Verification items for this drawing (mm, ordinates from the low corner). Round coordinates to 2 decimals unless told otherwise and drop trailing zeros. Order: outer loops, then holes, each group sorted by start corner. A loop starts at its lowest first (then second) coordinate and runs counter-clockwise, first axis right, second up. Notation, with made-up numbers: (74.25, 81.5) -> (105.25, 81.5) arc R26 cw to (105.25, 95.5) -> close; hole circle Ø8 at (-7, 34). An arc over 180 degrees is marked (long way). Return JSON: item names as keys, results as strings. Group by question number.
Item 1: Sectioned sample at C-C on y = 11. Record the cut outline in (x, z).
Item 2: Draft check along Z on the marked faces 1, 2 and 3. Enter one of: pulls with the +Z half, pulls with the -Z half, needs draft (parallel to the pull), parting line crosses it, or undercut.
Item 3: Depth check by flat-ended pin: pin 1 Ø2 at (x, y) = (44, 9) entering from +Z; pin 2 Ø8 at (x, z) = (81, 79.5) entering from -Y; pin 3 Ø23.5 at (x, z) = (45, 45) entering from -Y; pin 4 Ø3 at (x, z) = (58, 72) entering from -Y. Enter the tip coordinate at first touch or a pass-through.
Item 4: Sectioned sample at A-A on x = 45. Record the cut outline in (y, z).
Item 5: Sectioned sample at D-D on z = 14. Record the cut outline in (x, y).
Item 6: Scan lines: probe 1 along X at (y, z) = (26.45, 45); probe 2 along Y at (x, z) = (72, 51.5); probe 3 along X at (y, z) = (19.25, 45). Record each from-to range of solid material in increasing order. Write a range as from..to.
Item 7: Sectioned sample at B-B on z = 45. Record the cut outline in (x, y), plus the area to 3 significant figures.
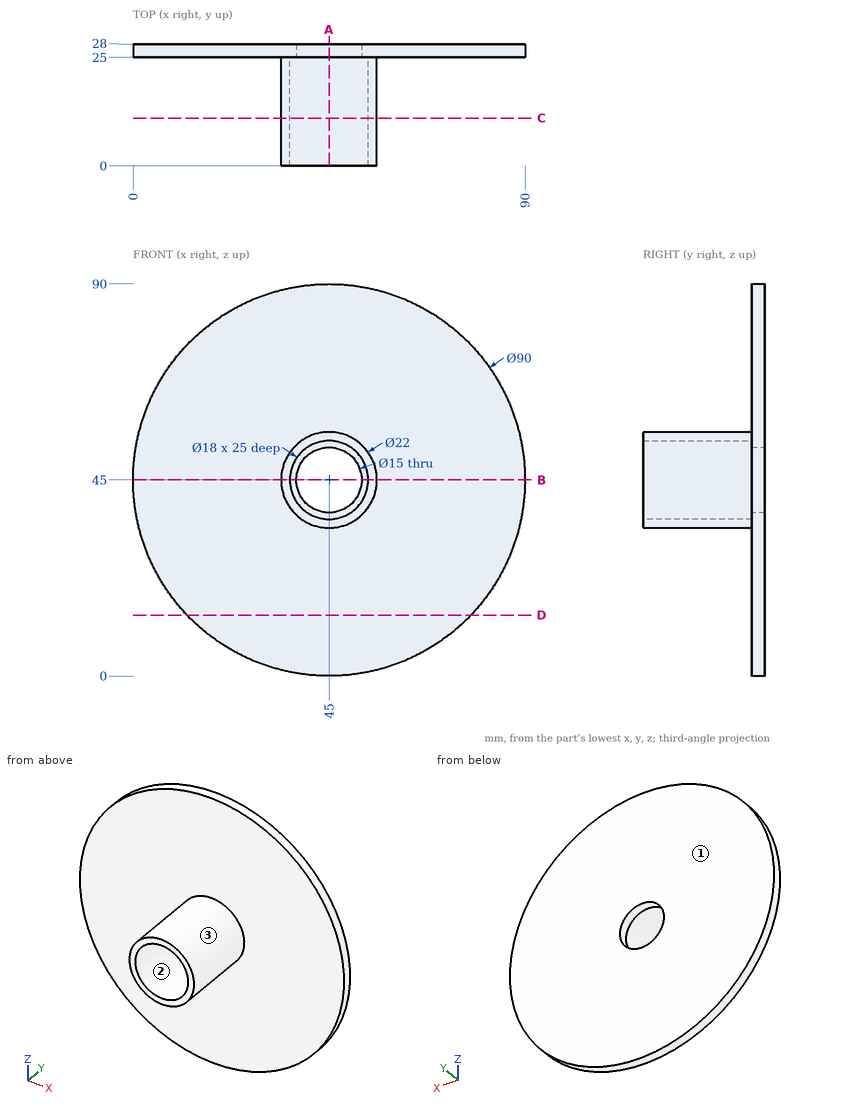
Recorded:
{
 "1": {"outline": "circle Ø22 at (45, 45); hole circle Ø18 at (45, 45)"},
 "2": {"face 1": "needs draft", "face 2": "undercut", "face 3": "parting line crosses it"},
 "3": {"pin 1": "z = 56", "pin 2": "through", "pin 3": "y = 0", "pin 4": "y = 25"},
 "4": {"outline": "(0, 34) -> (25, 34) -> (25, 0) -> (28, 0) -> (28, 37.5) -> (25, 37.5) -> (25, 36) -> (0, 36) -> close; (0, 54) -> (25, 54) -> (25, 52.5) -> (28, 52.5) -> (28, 90) -> (25, 90) -> (25, 56) -> (0, 56) -> close"},
 "5": {"outline": "(12.38, 25) -> (77.62, 25) -> (77.62, 28) -> (12.38, 28) -> close"},
 "6": {"probe 1": "0..37.5, 52.5..90", "probe 2": "25..28", "probe 3": "34..36, 54..56"},
 "7": {"outline": "(0, 25) -> (34, 25) -> (34, 0) -> (36, 0) -> (36, 25) -> (37.5, 25) -> (37.5, 28) -> (0, 28) -> close; (52.5, 25) -> (54, 25) -> (54, 0) -> (56, 0) -> (56, 25) -> (90, 25) -> (90, 28) -> (52.5, 28) -> close", "area": "325 mm²"}
}
